Geometry check sheet. Reference: drawing and pictorial views, mm from the part's lowest x, y, z. A direction names the side the tool comes from. Give positions to 0.01 mm unless a question says otherwise; leave off trailing zeros. Write each loop counter-clockwise with the first axis right and the second up, starting at its lowest first coordinate (ties: lowest second). Pieces come first, ordered by that corner, then holes. Notation, with made-up numbers: (6.5, 82) -> (43.5, 82) arc R19 ccw to (43.5, 100) -> close; hole circle Ø5 at (19, 27). An arc over 180 degrees is marked (long way). Return JSON: item names as keys, results as strings.
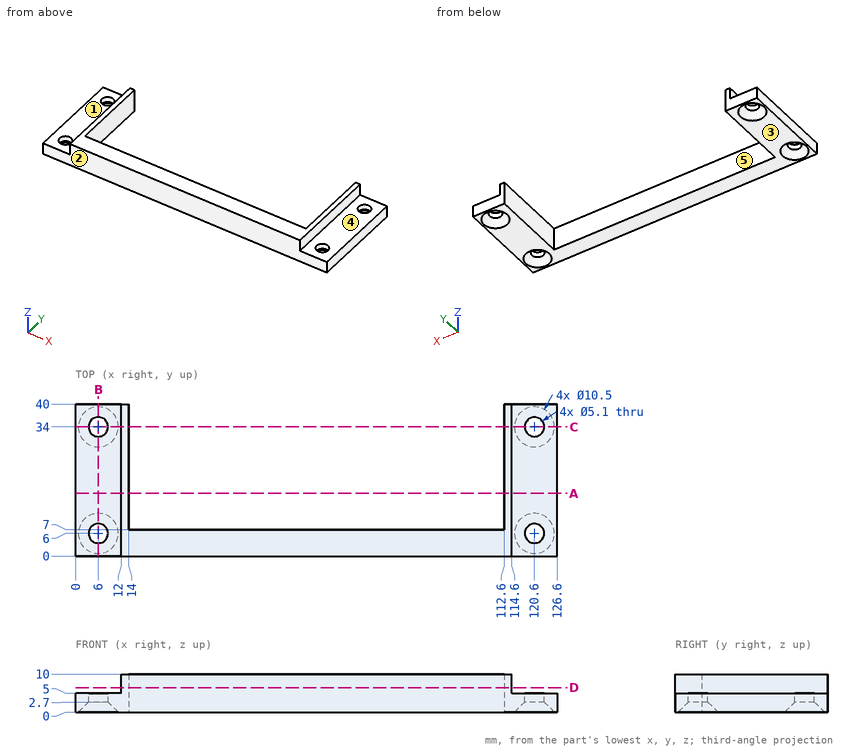
(1) Cross-section at B-B on x = 6. Enter the section's corners in (y, z).
Reply:
{"outline": "(0, 0) -> (0.75, 0) -> (3.45, 2.7) -> (3.45, 5) -> (0, 5) -> close; (8.55, 2.7) -> (11.25, 0) -> (28.75, 0) -> (31.45, 2.7) -> (31.45, 5) -> (8.55, 5) -> close; (36.55, 2.7) -> (39.25, 0) -> (40, 0) -> (40, 5) -> (36.55, 5) -> close"}
(2) Thickness scan on L1, parallel to Y at x = 6, z = 3.55; L2, parallel to X at y = 34, z = 3.9; L3, parallel to X at y = 6, z = 3.2. Record the ranges inside material, lowest first.
Reply:
{"L1": "0 to 3.45, 8.55 to 31.45, 36.55 to 40", "L2": "0 to 3.45, 8.55 to 14, 112.6 to 118.05, 123.15 to 126.6", "L3": "0 to 3.45, 8.55 to 118.05, 123.15 to 126.6"}
(3) Depth check by flat-ended pin: pin 1 Ø4.5 at (x, y) = (120.6, 34) entering from +Z; pin 2 Ø9.5 at (x, y) = (122.5, 12.5) entering from +Z; pin 3 Ø1 at (x, z) = (87, 2.5) entering from +Y; pin 4 Ø4 at (y, z) = (26, 8) entering from -X. Enter the tip coordinate at first touch or a pass-through.
Reply:
{"pin 1": "through", "pin 2": "z = 5", "pin 3": "y = 7", "pin 4": "x = 12"}
(4) Cross-section at D-D on z = 6.5. Enter the section's corners in (x, y), then the cut area to 3 significant figures.
Reply:
{"outline": "(12, 0) -> (114.6, 0) -> (114.6, 40) -> (112.6, 40) -> (112.6, 7) -> (14, 7) -> (14, 40) -> (12, 40) -> close", "area": "850 mm^2"}
(5) Set-up check for the marked faces 1, 2, 3, 4 and 5: record each of +Z, -Z, +X, -X, +Y, -Y from which the full face is reachable in a straight line by a thin tool's end or side.
Reply:
{"face 1": "+Z, -X, +Y, -Y", "face 2": "+Z, -Z, +X, -X, -Y", "face 3": "-Z, +X, -X, +Y, -Y", "face 4": "+Z, +X, +Y, -Y", "face 5": "+Z, -Z, +Y"}
(6) Cross-section at A-A on y = 16.5. Enter the section's corners in (x, z), then the cut area to 3 significant figures.
Reply:
{"outline": "(0, 0) -> (14, 0) -> (14, 10) -> (12, 10) -> (12, 5) -> (0, 5) -> close; (112.6, 0) -> (126.6, 0) -> (126.6, 5) -> (114.6, 5) -> (114.6, 10) -> (112.6, 10) -> close", "area": "160 mm^2"}
(7) Cross-section at C-C on y = 34. Enter the section's corners in (x, z), then the cut area to 3 significant figures.
Reply:
{"outline": "(0, 0) -> (0.75, 0) -> (3.45, 2.7) -> (3.45, 5) -> (0, 5) -> close; (8.55, 2.7) -> (11.25, 0) -> (14, 0) -> (14, 10) -> (12, 10) -> (12, 5) -> (8.55, 5) -> close; (112.6, 0) -> (115.35, 0) -> (118.05, 2.7) -> (118.05, 5) -> (114.6, 5) -> (114.6, 10) -> (112.6, 10) -> close; (123.15, 2.7) -> (125.85, 0) -> (126.6, 0) -> (126.6, 5) -> (123.15, 5) -> close", "area": "94.4 mm^2"}
